For this review, take the finished solid that the model builds, in its own axes (mm). A direction names the side the tool comes from. Give positions to 0.01 mm unless a question says otherwise; leave off trailing zeros. Write each loop counter-clockwise with the first axis right and the second up, starting at its lowest first coordinate (ties: lowest second). Pieces come first, ordered by that corner, then holes.
1) Wall thickness on line 1 along X through (y, z) = (3.5, 7.25); line 2 along X through (y, z) = (-22, 11); line 3 along Y through (x, z) = (-3, 13.75): over which ranges is each line inside the solid? List them lowest first.
2) Machinability: for faces 1 (the face through (-6, -1, 20)), 2 (the face through (7, 15.735, 3)), 3 (the face through (-13, -0.265, 10)), 4 (the face through (-11, -4.265, 12)), 5 (the face through (-0.686, 6, 12)), which of the approach directions +Z, -Z, +X, -X, +Y, -Y give a long, thin tool a straight path to every point of the face, cutting with its end or side? Answer none if there is none.
3) We need section D-D on x = -8. Give the boundary of the cut face in (y, z), and give its area (3 significant figures).
4) We need section C-C on x = -13. Give the boundary of the cut face in (y, z), and give its area (3 significant figures).
5) For P1, Ø3, axis at x = -11, z = 7.5, coming from the +Y side; P2, Ø12, axis at y = 1.5, z = 9, coming from the -X side; P3, Ø1, axis at x = -7.5, y = -8.5, coming from the +Z side; P4, Ø3, axis at x = 7.81, y = 8.24, coming from the +Z side, all flat-tipped, find the tip position at first contact; note any pin that passes through.
6) We need section A-A on z = 12.75. Give the boundary of the cut face in (x, y), and give its area (3 significant figures).
7) Draft analysis for pull direction X (two halves, no side actions). For faces 6 (the face through (-11, -21, 20)), 7 (the face through (18.314, -4, 10)), 8 (the face through (-0.686, -21, 13)), state which applies: pulls with the +X half, pulls with the -X half, needs draft (parallel to the pull), parting line crosses it, or undercut.
8) We need section B-B on y = 5. Give the boundary of the cut face in (x, z).
from build123d import *

# Parameters (mm, degrees)
BOSS_EXTRUDE1_DEPTH = 5
BOSS_EXTRUDE2_DEPTH = 20
SKETCH4_W           = 35
SKETCH4_H           = 4
BOSS_EXTRUDE3_DEPTH = 20
SKETCH6_R           = 1.8
CUT_EXTRUDE3_DEPTH  = 6
SKETCH7_W           = 4
SKETCH7_H           = 39
BOSS_EXTRUDE4_DEPTH = 20
SKETCH8_W           = 15
SKETCH8_H           = 15
CUT_EXTRUDE4_DEPTH  = 40


with BuildPart() as part:
    # Sketch1 → Boss-Extrude1 (new body)
    with BuildSketch(Plane.XY):
        Polygon((-20.68627451, -4.264705882), (-0.68627451, -4.264705882), (-0.68627451, 15.735294118), (14.31372549, 15.735294118), (14.31372549, -4.264705882), (14.31372549, -19.264705882), (-20.68627451, -19.264705882), align=None)
    extrude(amount=BOSS_EXTRUDE1_DEPTH)

    # Sketch2 → Boss-Extrude2 (add)
    with BuildSketch(Plane(origin=(0, 0, 0), x_dir=(-1, 0, 0), z_dir=(0, 0, -1))):
        Polygon((0.68627451, 15.735294118), (4.68627451, 15.735294118), (4.68627451, -0.264705882), (6.079970528, -0.264705882), (20.68627451, -0.264705882), (20.68627451, -4.264705882), (0.68627451, -4.264705882), align=None)
    extrude(amount=-BOSS_EXTRUDE2_DEPTH)

    # Sketch4 → Boss-Extrude3 (add)
    with BuildSketch(Plane(origin=(0, 0, 0), x_dir=(-1, 0, 0), z_dir=(0, 0, -1))):
        with Locations((3.18627451, -21.264705882)):
            Rectangle(SKETCH4_W, SKETCH4_H)
    extrude(amount=-BOSS_EXTRUDE3_DEPTH)

    # Sketch6 → Cut-Extrude3 (cut, through all)
    with BuildSketch(Plane.XY.offset(5)):
        with Locations((7.81372549, 8.235294118)):
            Circle(SKETCH6_R)
        with Locations((-13.18627451, -11.764705882)):
            Circle(SKETCH6_R)
    extrude(amount=-CUT_EXTRUDE3_DEPTH, mode=Mode.SUBTRACT)

    # Sketch7 → Boss-Extrude4 (add)
    with BuildSketch(Plane(origin=(0, 0, 0), x_dir=(-1, 0, 0), z_dir=(0, 0, -1))):
        with Locations((-16.31372549, -3.764705882)):
            Rectangle(SKETCH7_W, SKETCH7_H)
    extrude(amount=-BOSS_EXTRUDE4_DEPTH)

    # Sketch8 → Cut-Extrude4 (cut, through all)
    with BuildSketch(Plane(origin=(0, 15.735294118, 0), x_dir=(1, 0, 0), z_dir=(0, 1, 0))):
        with Locations((6.81372549, -12.5)):
            Rectangle(SKETCH8_W, SKETCH8_H)
    extrude(amount=-CUT_EXTRUDE4_DEPTH, mode=Mode.SUBTRACT)


solid = part.part
Results list:
1. line 1: x = -4.69 to -0.69, 14.31 to 18.31
1. line 2: x = -20.69 to -0.69, 14.31 to 18.31
1. line 3: y = -23.26 to -19.26, -4.26 to 15.74
2. face 1: +Z, +X, -X, +Y, -Y
2. face 2: +Z, -Z, +X, -X, +Y
2. face 3: +Z, -Z, -X, +Y
2. face 4: +Z, -X
2. face 5: +Z, +Y, -Y
3. outline: (-23.26, 0) - (-0.26, 0) - (-0.26, 20) - (-4.26, 20) - (-4.26, 5) - (-19.26, 5) - (-19.26, 20) - (-23.26, 20) - close
3. area: 235 mm2
4. outline: (-23.26, 0) - (-13.56, 0) - (-13.56, 5) - (-19.26, 5) - (-19.26, 20) - (-23.26, 20) - close; (-9.97, 0) - (-0.26, 0) - (-0.26, 20) - (-4.26, 20) - (-4.26, 5) - (-9.97, 5) - close
4. area: 217 mm2
5. P1: stops at y = -0.26
5. P2: stops at x = -20.69
5. P3: stops at z = 5
5. P4: passes through
6. outline: (-20.69, -23.26) - (-0.69, -23.26) - (-0.69, -19.26) - (-20.69, -19.26) - close; (-20.69, -4.26) - (-0.69, -4.26) - (-0.69, 15.74) - (-4.69, 15.74) - (-4.69, -0.26) - (-20.69, -0.26) - close; (14.31, -23.26) - (18.31, -23.26) - (18.31, 15.74) - (14.31, 15.74) - close
6. area: 380 mm2
7. face 6: needs draft
7. face 7: pulls with the +X half
7. face 8: undercut
8. outline: (-4.69, 0) - (18.31, 0) - (18.31, 20) - (14.31, 20) - (14.31, 5) - (-0.69, 5) - (-0.69, 20) - (-4.69, 20) - close
